from build123d import *

# Parameters (mm, degrees)
F1_DEPTH     = 20
F0_W         = 39.9660819769
F0_H         = 39.9660819769
F2_DEPTH     = 2
F4_DEPTH     = 20
F5_W         = 29.9660819769
F5_H         = 7.5
F6_DEPTH     = 3
F7_T4_DEPTH  = 66.2397385768
F8_W         = 29.9660819769
F8_H         = 7.5
F9_DEPTH     = 3
F10_T4_DEPTH = 66.2397385768
F11_DEPTH    = 1
F12_DEPTH    = 1
F13_SIZE     = 7


# Not quite as in the source:
# - a fillet or chamfer that OpenCascade refuses, or shapes differently, is made with other operations: its cross-section is extruded or revolved along the edge and cut away or added


with BuildPart() as f1:
    # F0 (on Top) → F1 (new body)
    with BuildSketch(Plane.XY):
        Polygon((24.9830409884, -24.9830409884), (24.9830409884, 19.9830409884), (19.9830409884, 19.9830409884), (19.9830409884, -19.9830409884), (-19.9830409884, -19.9830409884), (-19.9830409884, -24.9830409884), align=None)
        Polygon((24.9830409884, 24.9830409884), (-24.9830409884, 24.9830409884), (-24.9830409884, -24.9830409884), (-19.9830409884, -24.9830409884), (-19.9830409884, -19.9830409884), (-19.9830409884, 19.9830409884), (19.9830409884, 19.9830409884), (24.9830409884, 19.9830409884), align=None)
    extrude(amount=F1_DEPTH)

    # F0 (on Top) → F2 (join)
    with BuildSketch(Plane.XY):
        Polygon((24.9830409884, 24.9830409884), (-24.9830409884, 24.9830409884), (-24.9830409884, -24.9830409884), (-19.9830409884, -24.9830409884), (-19.9830409884, -19.9830409884), (-19.9830409884, 19.9830409884), (19.9830409884, 19.9830409884), (24.9830409884, 19.9830409884), align=None)
        Rectangle(F0_W, F0_H)
        Polygon((24.9830409884, -24.9830409884), (24.9830409884, 19.9830409884), (19.9830409884, 19.9830409884), (19.9830409884, -19.9830409884), (-19.9830409884, -19.9830409884), (-19.9830409884, -24.9830409884), align=None)
    extrude(amount=-F2_DEPTH)

    # F3 (on face) → F4 (join)
    with BuildSketch(Plane(origin=(0, 0, -2), x_dir=(1, 0, 0), z_dir=(0, 0, -1))):
        Polygon((24.9830409884, -24.9830409884), (24.9830409884, 19.9830409884), (19.9830409884, 19.9830409884), (19.9830409884, -19.9830409884), (-19.9830409884, -19.9830409884), (-19.9830409884, -24.9830409884), align=None)
    extrude(amount=F4_DEPTH)

    # F5 (on face) → F6 (join)
    with BuildSketch(Plane(origin=(-24.9830409884, 0, 0), x_dir=(0, -1, 0), z_dir=(-1, 0, 0))):
        with Locations((0, 1.75)):
            Rectangle(F5_W, F5_H)
        with Locations((0, -5.75)):
            Rectangle(F5_W, F5_H)
    extrude(amount=F6_DEPTH)

    # F7: chamfer of 7 x 3.2641536071 on 1 edges, made by hand


with BuildPart() as f7_tool2:
    # F7_s3 → F7_t4 (new body)
    with BuildSketch(Plane.XZ.offset(33.1198692884)):
        Polygon((-24.7188873814, 5.5), (-27.9830409884, -1.5), (-27.9830409884, 5.5), align=None)
    extrude(amount=-F7_T4_DEPTH)

    split(bisect_by=Plane.YZ.offset(-24.9830409884), keep=Keep.BOTTOM)


with BuildPart() as f1_1:
    add(f1.part)

    # F7_t1: cut F7_tool2
    add(f7_tool2.part, mode=Mode.SUBTRACT)

    # F8 (on face) → F9 (join)
    with BuildSketch(Plane.XZ.offset(24.9830409884)):
        with Locations((0, 1.75)):
            Rectangle(F8_W, F8_H)
        with Locations((0, -5.75)):
            Rectangle(F8_W, F8_H)
    extrude(amount=F9_DEPTH)

    # F10: chamfer of 7 x 3.2641536071 on 1 edges, made by hand


with BuildPart() as f10_tool2:
    # F10_s3 → F10_t4 (new body)
    with BuildSketch(Plane.YZ.offset(33.1198692884)):
        Polygon((-24.7188873814, 5.5), (-27.9830409884, -1.5), (-27.9830409884, 5.5), align=None)
    extrude(amount=-F10_T4_DEPTH)

    split(bisect_by=Plane.XZ.offset(24.9830409884), keep=Keep.TOP)


with BuildPart() as f1_2:
    add(f1_1.part)

    # F10_t1: cut F10_tool2
    add(f10_tool2.part, mode=Mode.SUBTRACT)

    # F11 (add): a face of the model
    f11_faces = [f1_2.faces().sort_by_distance(p)[0] for p in [
        (0, -24.9830409884, -5.75),
    ]]
    extrude(f11_faces, amount=F11_DEPTH)

    # F12 (add): a face of the model
    f12_faces = [f1_2.faces().sort_by_distance(p)[0] for p in [
        (-24.9830409884, 0, -5.75),
    ]]
    extrude(f12_faces, amount=F12_DEPTH)

    # F13
    f13_edges = [f1_2.edges().sort_by_distance(p)[0] for p in [
        (-24.983041, -24.983041, 9),
    ]]
    chamfer(f13_edges, length=F13_SIZE)


solid = f1_2.part
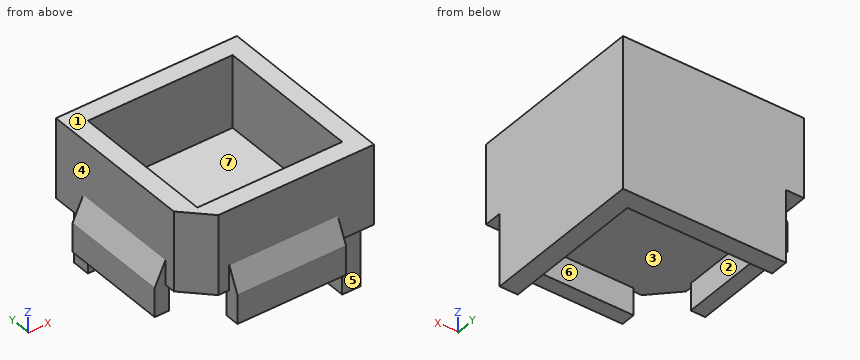
The model under review builds one solid part; all positions refer to its coordinate system, in mm. Face numbers are marked on the shaded views. A direction names the side the tool comes from. Coordinates: 2 decimals unless noted, no trailing zeros. Write each loop counter-clockwise with the first axis right and the second up, starting at its lowest first coordinate (ties: lowest second). Pieces come first, ordered by that corner, then holes. Notation, with made-up numbers: M 84.5,87 L 102.5,87 A20 cw 102.5,93 Z; hole C -16,88.25 d3. An arc over 180 degrees is marked long. Put each result on its own line as item: value.
1) Wall thickness on probe 1 along Y at (x, z) = (-1, 17.5); probe 2 along Z at (x, y) = (-9, 0.5): over which ranges is each line inside the solid? List them lowest first. Write a range as [from, to].
Computed:
probe 1: y = [-24.98, -19.98], [19.98, 24.98]
probe 2: z = [-2, 0]
2) Clearance check with flat-ended pins moving along their axes: pin 1 Ø10 at (y, z) = (8.5, 13.5) entering from -X; pin 2 Ø22 at (x, z) = (2.5, 13.5) entering from -Y; pin 3 Ø6 at (x, z) = (-2, 15) entering from -Y. State where each tip first meets the part, or that it passes through.
Computed:
pin 1: stops at x = -24.98
pin 2: stops at y = -26.12
pin 3: stops at y = -24.98
3) For the marked faces 5, 6 and 7, list the 3-axis set-ups (+Z, -Z, +X, -X, +Y, -Y) from which the entire face can be reached by the end or side of a thin tool; tool diameter is ignored.
Computed:
face 5: -Z, +X, -X, -Y
face 6: -Z, +X, -X
face 7: +Z
4) Add section B-B on y = -10. Give the boundary of the cut face in (x, z).
Computed:
outline: M -27.98,-9.5 L -23.98,-9.5 L -23.98,-2 L 19.98,-2 L 19.98,-22 L 24.98,-22 L 24.98,20 L 19.98,20 L 19.98,0 L -19.98,0 L -19.98,20 L -24.98,20 L -24.98,4.93 L -27.98,-1.5 Z
5) Add section A-A on z = -8.5. Give the boundary of the cut face in (x, y), then the cut area to 3 significant figures.
Computed:
outline: M -27.98,-14.98 L -23.98,-14.98 L -23.98,14.98 L -27.98,14.98 Z; M -19.98,19.98 L 19.98,19.98 L 19.98,-19.98 L 24.98,-19.98 L 24.98,24.98 L -19.98,24.98 Z; M -14.98,-27.98 L 14.98,-27.98 L 14.98,-23.98 L -14.98,-23.98 Z
area: 664 mm2
6) Add section D-D on z = 12. Give the boundary of the cut face in (x, y).
Computed:
outline: M -24.98,-17.98 L -17.98,-24.98 L 24.98,-24.98 L 24.98,24.98 L -24.98,24.98 Z; hole M -19.98,-19.98 L 19.98,-19.98 L 19.98,19.98 L -19.98,19.98 Z
7) Draft analysis for pull direction X (two halves, no side actions). For the marked faces 1, 2, 3 and 4, state which applies: released by +X, released by -X, zero draft, split by the parting line, or undercut.
Computed:
face 1: zero draft
face 2: undercut
face 3: undercut
face 4: released by -X
